Verification items for this drawing (mm, ordinates from the low corner). A direction names the side the tool comes from. Coordinates: 2 decimals unless noted, no trailing zeros. Write each loop counter-clockwise with the first axis right and the second up, starting at its lowest first coordinate (ties: lowest second). Pieces come first, ordered by that corner, then holes. Notation, with made-up numbers: (47.25, 81.5) -> (68.25, 81.5) arc R12 ccw to (68.25, 102.5) -> close; hole circle Ø2 at (4, -8). An arc over 180 degrees is marked (long way). One line per item, written item: value. Start each with the question number.
1) Sectioned sample at A-A on x = 4. Enter the section's corners in (y, z).
2) Gauge pin test, flat ends, axial feed: P1, Ø1, axis at y = 18, z = 5, coming from the -X side; P2, Ø3, axis at x = 2, y = 9.5, coming from the +Z side (1 decimal); P3, Ø1.5, axis at x = 3, y = 11.5, coming from the -Z side (1 decimal). Record the tip position at first contact, or that the pin passes through.
3) Scan lines: line 1 along Y through (x, z) = (4, 1.25); line 2 along X through (y, z) = (3.5, 3); line 3 along X through (y, z) = (1.25, 2.5). Record each from-to range of solid material in increasing order. Write a range as [from, to].
4) Sectioned sample at D-D on x = 8.25. Enter the section's corners in (y, z), plus the area to 3 significant figures.
5) Sectioned sample at B-B on z = 5. Enter the section's corners in (x, y), plus the area to 3 significant figures.
6) Sectioned sample at C-C on y = 13.25. Enter the section's corners in (x, z).
7) Set-up check for the marked faces 1 and 2: record each of +Z, -Z, +X, -X, +Y, -Y from which the full face is reachable in a straight line by a thin tool's end or side.
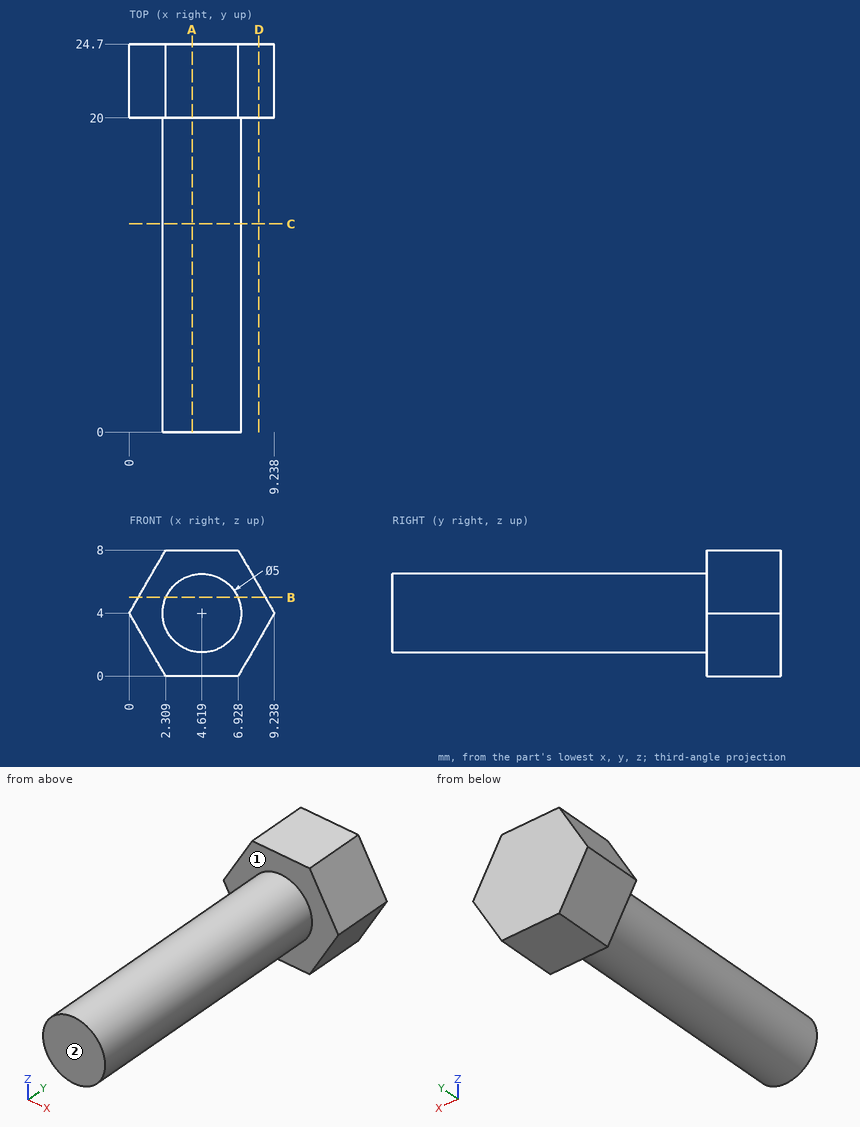
Answers:
1. outline: (0, 1.58) -> (20, 1.58) -> (20, 0) -> (24.7, 0) -> (24.7, 8) -> (20, 8) -> (20, 6.42) -> (0, 6.42) -> close
2. P1: stops at x = 2.17
2. P2: stops at z = 6.2
2. P3: stops at z = 1.7
3. line 1: y = [20, 24.7]
3. line 2: x = [2.33, 6.91]
3. line 3: x = [2.62, 6.62]
4. outline: (20, 2.29) -> (24.7, 2.29) -> (24.7, 5.71) -> (20, 5.71) -> close
4. area: 16.1 mm2
5. outline: (0.58, 20) -> (2.33, 20) -> (2.33, 0) -> (6.91, 0) -> (6.91, 20) -> (8.66, 20) -> (8.66, 24.7) -> (0.58, 24.7) -> close
5. area: 130 mm2
6. outline: circle Ø5 at (4.62, 4)
7. face 1: -Y
7. face 2: +Z, -Z, +X, -X, -Y
